Model file for the job. Use its own axes, mm. Face numbers are marked on the shaded views. A direction names the side the tool comes from. Give positions to 0.01 mm unless a question says otherwise; leave off trailing zeros. Write each loop counter-clockwise with the first axis right and the second up, starting at its lowest first coordinate (ties: lowest second). Pieces come first, ordered by that corner, then holes.
```python
from build123d import *

# Parameters (mm, degrees)
SKETCH1_R           = 2
BOSS_EXTRUDE1_DEPTH = 30
SKETCH2_R           = 4.75
BOSS_EXTRUDE2_DEPTH = 2
CHAMFER1_SIZE       = 1.7


with BuildPart() as part:
    # Sketch1 → Boss-Extrude1 (new body)
    with BuildSketch(Plane(origin=(0, 0, 0), x_dir=(1, 0, 0), z_dir=(0, 1, 0))):
        with Locations(Location((0, 0, 0), (0, 0, 270))):
            Circle(SKETCH1_R)
    extrude(amount=BOSS_EXTRUDE1_DEPTH)

    # Sketch2 → Boss-Extrude2 (add)
    with BuildSketch(Plane(origin=(0, 30, 0), x_dir=(1, 0, 0), z_dir=(0, 1, 0))):
        with Locations(Location((0, 0, 0), (0, 0, 270))):
            Circle(SKETCH2_R)
    extrude(amount=BOSS_EXTRUDE2_DEPTH)

    # Chamfer1
    chamfer1_edges = [part.edges().sort_by_distance(p)[0] for p in [
        (0, 32, -4.75),
    ]]
    chamfer(chamfer1_edges, length=CHAMFER1_SIZE)


solid = part.part
```
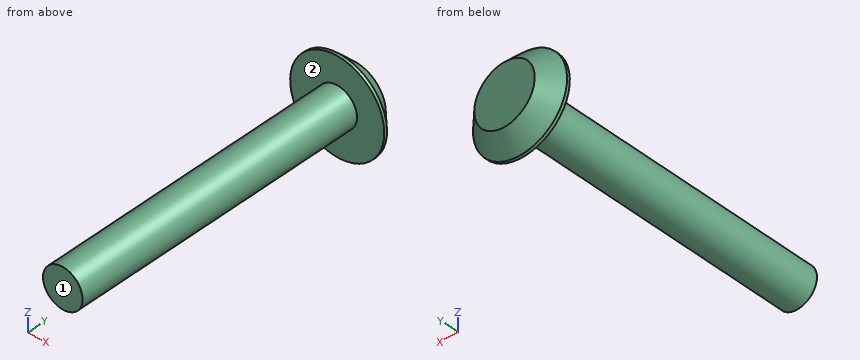
1. Slice it at A-A, the plane x = 0. Write the cut outline in (y, z), and give its area (3 significant figures).
Calculated:
outline: (0, -2) - (30, -2) - (30, -4.75) - (30.3, -4.75) - (32, -3.05) - (32, 3.05) - (30.3, 4.75) - (30, 4.75) - (30, 2) - (0, 2) - close
area: 136 mm2
2. Which spindle directions (+Z, -Z, +X, -X, +Y, -Y) get a long thin tool onto all of the face, cutting with end or side? Do the marked faces 1 and 2. Say none if no direction does.
Calculated:
face 1: +Z, -Z, +X, -X, -Y
face 2: -Y
3. Probe probe 1 along Y at (x, z) = (-2.5, 1.5); probe 2 along Z at (x, y) = (1.5, 17.5); probe 3 along Y at (x, z) = (-2.5, -2). List the from-to ranges inside material, lowest first.
Calculated:
probe 1: y = 30 to 32
probe 2: z = -1.32 to 1.32
probe 3: y = 30 to 31.85
4. Pin check, flat tips, straight feed: P1, Ø2, axis at x = -1, z = -1, coming from the -Y side; P2, Ø3, axis at y = 20, z = -3, coming from the -X side; P3, Ø1.5, axis at y = 12, z = -2.5, coming from the -X side; P4, Ø5, axis at y = 5, z = -2.5, coming from the -X side. Stop position of each tip, or through.
Calculated:
P1: stops at y = 0
P2: stops at x = -1.32
P3: stops at x = -0.97
P4: stops at x = -2
5. Slice it at C-C, the plane y = 20.5. Write the cut outline in (x, z), and give its area (3 significant figures).
Calculated:
outline: circle Ø4 at (0, 0)
area: 12.6 mm2
6. Slice it at B-B, the plane z = 0. Write the cut outline in (x, y).
Calculated:
outline: (-4.75, 30) - (-2, 30) - (-2, 0) - (2, 0) - (2, 30) - (4.75, 30) - (4.75, 30.3) - (3.05, 32) - (-3.05, 32) - (-4.75, 30.3) - close
